from build123d import *

# Parameters (mm, degrees)
F1_DEPTH = 25


# Not quite as in the source:
# - the program builds the solid bodies; features that only make, move or delete a surface that nothing else refers to are left out


with BuildPart() as f1:
    # F0 (on Front) → F1 (new body)
    with BuildSketch(Plane.XZ):
        with BuildLine():
            ThreePointArc((-20, -34.6410161514), (-10.3527618041, -38.6370330516), (0, -40))
            Line((0, -40), (0, -36.5303086516))
            add(Edge.make_bspline(
                [(0, -36.5303086516), (-0.1149220611, -36.5363907695), (-0.234185262, -36.5363907695)],
                knots=[0.9158257876, 0.9158257876, 0.9158257876, 1, 1, 1], degree=2))
            add(Edge.make_bspline(
                [(-0.234185262, -36.5363907695), (-1.8148580784, -36.5363907695), (-2.6530614293, -35.3588639809)],
                knots=[0, 0, 0, 1, 1, 1], degree=2))
            add(Edge.make_bspline(
                [(-2.6530614293, -35.3588639809), (-3.4912647801, -34.1813371924), (-3.4912647801, -31.9347820187)],
                knots=[0, 0, 0, 1, 1, 1], degree=2))
            add(Edge.make_bspline(
                [(-3.4912647801, -31.9347820187), (-3.4912647801, -29.5010139137), (-2.6200864243, -28.1979693646)],
                knots=[0, 0, 0, 1, 1, 1], degree=2))
            add(Edge.make_bspline(
                [(-2.6200864243, -28.1979693646), (-1.7489080686, -26.8949248154), (-0.1405787965, -26.8949248154)],
                knots=[0, 0, 0, 1, 1, 1], degree=2))
            add(Edge.make_bspline(
                [(-0.1405787965, -26.8949248154), (-0.0694054692, -26.8949248154), (0, -26.8970735535)],
                knots=[0, 0, 0, 0.0335559038, 0.0335559038, 0.0335559038], degree=2))
            Line((0, -26.8970735535), (0, 0))
            Line((0, 0), (-14.4835999879, -25.0863310555))
            Line((-14.4835999879, -25.0863310555), (-12.9261437307, -25.0863310555))
            Line((-12.9261437307, -25.0863310555), (-12.9261437307, -26.0823037829))
            add(Edge.make_bspline(
                [(-12.9261437307, -26.0823037829), (-14.4004454653, -28.334163173), (-15.0087314402, -29.6107992676)],
                knots=[0, 0, 0, 1, 1, 1], degree=2))
            add(Edge.make_bspline(
                [(-15.0087314402, -29.6107992676), (-15.6170174151, -30.8874353622), (-15.9206143649, -32.1302171206)],
                knots=[0, 0, 0, 1, 1, 1], degree=2))
            add(Edge.make_bspline(
                [(-15.9206143649, -32.1302171206), (-16.2242113147, -33.3729988791), (-16.2242113147, -34.7031466663)],
                knots=[0, 0, 0, 1, 1, 1], degree=2))
            Line((-16.2242113147, -34.7031466663), (-17.5063077861, -34.7031466663))
            add(Edge.make_bspline(
                [(-17.5063077861, -34.7031466663), (-17.5063077861, -32.8597234604), (-16.7254739044, -30.823002916)],
                knots=[0, 0, 0, 1, 1, 1], degree=2))
            add(Edge.make_bspline(
                [(-16.7254739044, -30.823002916), (-15.9446400228, -28.7862823716), (-14.1143217212, -26.1303550987)],
                knots=[0, 0, 0, 1, 1, 1], degree=2))
            Line((-14.1143217212, -26.1303550987), (-15.0863675502, -26.1303550987))
            Line((-15.0863675502, -26.1303550987), (-20, -34.6410161514))
        make_face()
    extrude(amount=F1_DEPTH)


solid = f1.part
Input: part model. Units: mm. Frame: model coordinates. A direction names the side the tool comes from. Give positions to 0.01 mm unless a question says otherwise; leave off trailing zeros. Order: outer loops, then holes, each group sorted by start corner. A loop starts at its lowest first (then second) coordinate and runs counter-clockwise, first axis right, second up. Notation, with made-up numbers: M -4.75,-7.5 L 34.25,-7.5 A26 cw 34.25,21.5 Z; hole C -39,-16.75 d7. An arc over 180 degrees is marked long. Answer as a JSON object with one key per item and string values.
1. First-contact query: P1, Ø8, axis at y = -6.5, z = -16.5, coming from the -X side; P2, Ø1.4, axis at x = -17, y = -18, coming from the +Z side; P3, Ø1, axis at x = -16.5, y = -17.5, coming from the -Z side; P4, Ø1.5, axis at y = -5, z = -18, coming from the +X side. Flat tips, straight axial feed; report the tip coordinate or a pass-through.
Result sheet:
{"P1": "x = -11.84", "P2": "z = -28.23", "P3": "z = -36.66", "P4": "x = 0"}
2. Reachability of faces 5 (the flat face through (-14.6, -12.3, -26.13)), 6 (the flat face through (-17.51, -12.32, -30.33)) from +Z, -Z, +X, -X, +Y, -Y: full face, straight path, thin tool, end or side. Return the list, or none.
Result sheet:
{"face 5": "-X, +Y, -Y", "face 6": "+Z, -X, +Y, -Y"}
3. Ray query, line 1 (Z direction, x = -14.75, y = -20.5); line 2 (X direction, y = -1.75, z = -29); line 3 (X direction, y = -19, z = -30). Return the intervals inside material, ascending. Write a range as [from, to].
Result sheet:
{"line 1": "[-37.18, -29.1], [-27.08, -26.13]", "line 2": "[-16.74, -15.88], [-14.7, -3.03]", "line 3": "[-17.32, -16.38], [-15.19, -3.32]"}
4. Cut plane B-B, the plane x = -8.75. Output: boundary loops of the cut face in (y, z), and give its area (3 significant figures).
Result sheet:
{"outline": "M -25,-39.03 L 0,-39.03 L 0,-15.16 L -25,-15.16 Z", "area": "597 mm²"}
5. Cut plane A-A, the plane z = -16. Output: boundary loops of the cut face in (x, y), and give its area (3 significant figures).
Result sheet:
{"outline": "M -9.24,-25 L 0,-25 L 0,0 L -9.24,0 Z", "area": "231 mm²"}
6. Pull-direction query (X, two-part tool) for faces 1 (the flat face through (-12.926, -12.3, -25.6)), 2 (the flat face through (-17, -12, -34.703)), 3 (the flat face through (0, -12, -38)), 4 (the flat face through (-14, -12, -25.086)); classes: +X half, -X half, draft (parallel to the pull), parting line (faces both ways), or undercut.
Result sheet:
{"face 1": "-X half", "face 2": "undercut", "face 3": "+X half", "face 4": "draft"}
